Geometry check sheet. Reference: the model listing, model coordinates, mm. A direction names the side the tool comes from. Give positions to 0.01 mm unless a question says otherwise; leave off trailing zeros. Write each loop counter-clockwise with the first axis right and the second up, starting at its lowest first coordinate (ties: lowest second). Pieces come first, ordered by that corner, then holes. Notation, with made-up numbers: M 2.5,27.5 L 44.5,27.5 A6 cw 44.5,31.5 Z; hole C 19.25,81 d6. An arc over 180 degrees is marked long. One line per item, written item: value. Start each with the question number.
1. Cross-section at A-A on z = 7.25. Record the cut outline in (x, y), then the cut area to 3 significant figures.
2. Cross-section at B-B on x = 7.5. Record the cut outline in (y, z).
3. Scan lines: line 1 (Y direction, x = 12, z = 7.4); line 2 (Z direction, x = 8.75, y = 14.75). Record each from-to range of solid material in increasing order.
4. Release check for a two-part mould opening along X. For faces 1 (the face through (6, 6, 8)), 2 (the face through (13, 9, 4)), 3 (the face through (11, 8.9, 7.5)) record: pulls with the +X half, pulls with the -X half, needs draft (parallel to the pull), parting line crosses it, or undercut.
5. Cross-section at C-C on y = 7.5. Record the cut outline in (x, z), then the cut area to 3 significant figures.
6. Tool access check on faces 4 (the face through (6, 0, 4)), 5 (the face through (6.5, 4, 7.5)). Record the directions out of +Z, -Z, +X, -X, +Y, -Y that give a thin tool (end or side, any length) a straight path to the whole face; none if there is none.
7. Cross-section at D-D on y = 2.75. Record the cut outline in (x, z), then the cut area to 3 significant figures.
8. Gauge pin test, flat end, axial feed: pin 1 (0.8 mm diameter, centred on x = 12, y = 1, fed in from +Z). Record the tip position at first contact, or that the pin passes through.
from build123d import *

# Parameters (mm, degrees)
ESQUISSE1_W             = 13
ESQUISSE1_H             = 18
BOSS_EXTRU_1_DEPTH      = 8
ESQUISSE2_R             = 0.5
ESQUISSE2_W             = 9
ESQUISSE2_H             = 14
ESQUISSE2_W_2           = 5
ESQUISSE2_H_2           = 4
ENL_V_MAT_EXTRU_1_DEPTH = 1


with BuildPart() as part:
    # Esquisse1 → Boss.-Extru.1 (new body)
    with BuildSketch(Plane.XY):
        with Locations((6.5, 9)):
            Rectangle(ESQUISSE1_W, ESQUISSE1_H)
    extrude(amount=BOSS_EXTRU_1_DEPTH)

    # Esquisse2 → Enlèv. mat.-Extru.1 (cut)
    with BuildSketch(Plane.XY.offset(8)):
        with Locations((12, 1)):
            Circle(ESQUISSE2_R)
        with Locations((6.5, 9)):
            Rectangle(ESQUISSE2_W, ESQUISSE2_H)
        with Locations((6.5, 12)):
            Rectangle(ESQUISSE2_W_2, ESQUISSE2_H_2, mode=Mode.SUBTRACT)
        with Locations((6.5, 6)):
            Rectangle(ESQUISSE2_W_2, ESQUISSE2_H_2, mode=Mode.SUBTRACT)
    extrude(amount=-ENL_V_MAT_EXTRU_1_DEPTH, mode=Mode.SUBTRACT)


solid = part.part
Report:
1. outline: M 0,0 L 13,0 L 13,18 L 0,18 Z; M 4,4 L 9,4 L 9,8 L 4,8 Z; M 4,10 L 9,10 L 9,14 L 4,14 Z; hole M 2,2 L 11,2 L 11,16 L 2,16 Z; hole C 12,1 d1
1. area: 147 mm^2
2. outline: M 0,0 L 18,0 L 18,8 L 16,8 L 16,7 L 14,7 L 14,8 L 10,8 L 10,7 L 8,7 L 8,8 L 4,8 L 4,7 L 2,7 L 2,8 L 0,8 Z
3. line 1: y = 0 to 0.5, 1.5 to 18
3. line 2: z = 0 to 7
4. face 1: needs draft
4. face 2: pulls with the +X half
4. face 3: undercut
5. outline: M 0,0 L 13,0 L 13,8 L 11,8 L 11,7 L 9,7 L 9,8 L 4,8 L 4,7 L 2,7 L 2,8 L 0,8 Z
5. area: 100 mm^2
6. face 4: +Z, -Z, +X, -X, -Y
6. face 5: +Z
7. outline: M 0,0 L 13,0 L 13,8 L 11,8 L 11,7 L 2,7 L 2,8 L 0,8 Z
7. area: 95.0 mm^2
8. pin 1: stops at z = 7
